Build history of the part. All positions in model axes, mm. A direction names the side the tool comes from. Give positions to 0.01 mm unless a question says otherwise; leave off trailing zeros. Loops run counter-clockwise (first coordinate to the right, second up) from the corner with the lowest first, then second, coordinate; pieces in that order, holes last. Notation, with made-up numbers: M -18.5,22 L -5.5,22 A18 ccw -5.5,34 Z; hole C 75.5,59 d1. An arc over 180 degrees is marked long. Answer as a JSON object with one key per item and string values. Group by question number.
1. Slice it at C-C (y = 0). List the corners of the cut face in (x, z).
2. Drill centre lines: line 1 along Z through (x, y) = (-151, -150.5); line 2 along Z through (x, y) = (-277, 366); line 3 along Y through (x, z) = (0, -487). Where is each one in solid material? Low to high. Write a range as [from, to].
3. Slice it at D-D (z = -356). List the corners of the cut face in (x, y), then the cut area to 3 significant figures.
4. Slice it at A-A (y = 197). List the corners of the cut face in (x, z).
5. Drop a flat-ended pin along its axis: pin 1 Ø1 at (x, y) = (-1.5, -415.5) entering from -Z. Give the stop position or say it passes through.
6. Slice it at B-B (x = -95.5). List the corners of the cut face in (y, z), then the cut area to 3 significant figures.
7. 3-axis set-ups, long thin cutter, end or side, ignore diameter. For faces 4 (the face through (-55.55, 42.594, -345.1)), 5 (the face through (-8, 8, 20)): which of +Z, -Z, +X, -X, +Y, -Y reach the whole face in a straight line?
8. Mould opens along Z. For faces 1 (the face through (-4, -4, -720)), 2 (the face through (-8, -115, 0)), 3 (the face through (262.3, -82.6, -709.9)) say: released by +Z, released by -Z, zero draft, split by the parting line, or undercut.
from build123d import *

# Parameters (mm, degrees)
F0_R     = 550
F1_DEPTH = 20
F2_R     = 70
F3_DEPTH = 700
F4_R     = 275
F5_DEPTH = 20


with BuildPart() as f1:
    # F0 (on Top) → F1 (new body)
    with BuildSketch(Plane.XY):
        Circle(F0_R)
    extrude(amount=F1_DEPTH)

    # F2 (on face) → F3 (join)
    with BuildSketch(Plane(origin=(0, 0, 0), x_dir=(1, 0, 0), z_dir=(0, 0, -1))):
        Circle(F2_R)
    extrude(amount=F3_DEPTH)

    # F4 (on face) → F5 (join)
    with BuildSketch(Plane(origin=(0, 0, -700), x_dir=(1, 0, 0), z_dir=(0, 0, -1))):
        Circle(F4_R)
    extrude(amount=F5_DEPTH)


solid = f1.part
Established:
{
 "1": {"outline": "M -550,0 L -70,0 L -70,-700 L -275,-700 L -275,-720 L 275,-720 L 275,-700 L 70,-700 L 70,0 L 550,0 L 550,20 L -550,20 Z"},
 "2": {"line 1": "z = [-720, -700], [0, 20]", "line 2": "z = [0, 20]", "line 3": "y = [-70, 70]"},
 "3": {"outline": "C 0,0 d140", "area": "15,400 mm^2"},
 "4": {"outline": "M -513.51,0 L 513.51,0 L 513.51,20 L -513.51,20 Z; M -191.87,-720 L 191.87,-720 L 191.87,-700 L -191.87,-700 Z"},
 "5": {"pin 1": "stops at z = 0"},
 "6": {"outline": "M -541.65,0 L 541.65,0 L 541.65,20 L -541.65,20 Z; M -257.89,-720 L 257.89,-720 L 257.89,-700 L -257.89,-700 Z", "area": "32,000 mm^2"},
 "7": {"face 4": "none", "face 5": "+Z, +X, -X, +Y, -Y"},
 "8": {"face 1": "released by -Z", "face 2": "undercut", "face 3": "zero draft"}
}
